Could you check a few things on this model? Use its own coordinates, in mm. A direction names the side the tool comes from. Round coordinates to 2 decimals unless told otherwise and drop trailing zeros. Order: outer loops, then holes, each group sorted by start corner. A loop starts at its lowest first (then second) coordinate and runs counter-clockwise, first axis right, second up. Notation, with made-up numbers: (-2, 7) -> (5, 7) arc R8 ccw to (5, 13) -> close; hole circle Ø1 at (4, -23.5). An arc over 180 degrees is marked (long way). Put each result on its own line as item: value. Start each with the question number.
from build123d import *

# Parameters (mm, degrees)
SKETCH2_R           = 3
BOSS_EXTRUDE1_DEPTH = 30


with BuildPart() as part:
    # Sketch1 → Revolve1 (revolve)
    with BuildSketch(Plane.XY):
        Polygon((0, 0), (10, 0), (10, 1), (5, 1), (5, 4), (10, 4), (10, 5), (0, 5), align=None)
    revolve(axis=Axis((0, 5, 0), (0, -1, 0)))

    # Sketch2 → Boss-Extrude1 (add)
    with BuildSketch(Plane(origin=(0, 5, 0), x_dir=(1, 0, 0), z_dir=(0, 1, 0))):
        Circle(SKETCH2_R)
    extrude(amount=BOSS_EXTRUDE1_DEPTH)


solid = part.part
1. For pin 1 Ø4 at (x, y) = (4, 16) entering from -Z; pin 2 Ø2 at (y, z) = (21.5, 0.5) entering from -X; pin 3 Ø4 at (y, z) = (18, 4.5) entering from +X, each with a flat end and sliding along its axis, tell me the tip position at first contact or that it passes through.
2. If we section it at A-A, the plane x = -8: Please give me the cut outline in (y, z).
3. Thinking about a two-plate mould opening in Y: for faces 4 (the face through (-2.17, 4.51, -9.76)), 5 (the face through (2, 1, 5)), 6 (the face through (0, 0, 0)), which applies, +Y half, -Y half, draft (parallel to the pull), parting line (faces both ways), or undercut?
4. I need wall thicknesses on L1, parallel to Y at x = 6.5, z = 3.75; L2, parallel to Y at x = 4, z = 1; L3, parallel to X at y = 21, z = -1.5. Which ranges of each line are inside material? Lowest first, please.
5. Which directions (+Z, -Z, +X, -X, +Y, -Y) give clear straight access to the entire face, cutting with the end or side of a thin tool? Please do faces 1 (the face through (-1.08, 2.52, -4.88)), 2 (the face through (0, 35, 0)), 3 (the face through (2.1, 5, 2.4)).
6. If we section it at D-D, the plane x = 0: Please give me the cut outline in (y, z), then the cut area to 3 significant figures.
7. If we section it at B-B, the plane z = -5.75: Please give me the cut outline in (x, y), then the cut area to 3 significant figures.
8. If we section it at C-C, the plane z = 0: Please give me the cut outline in (x, y), then the cut area to 3 significant figures.
Results below:
1. pin 1: z = -2.24
1. pin 2: x = -3
1. pin 3: x = 1.66
2. outline: (0, -6) -> (1, -6) -> (1, 6) -> (0, 6) -> close; (4, -6) -> (5, -6) -> (5, 6) -> (4, 6) -> close
3. face 4: draft
3. face 5: undercut
3. face 6: -Y half
4. L1: 0 to 1, 4 to 5
4. L2: 0 to 5
4. L3: -2.6 to 2.6
5. face 1: none
5. face 2: +Z, -Z, +X, -X, +Y
5. face 3: +Y
6. outline: (0, -10) -> (1, -10) -> (1, -5) -> (4, -5) -> (4, -10) -> (5, -10) -> (5, -3) -> (35, -3) -> (35, 3) -> (5, 3) -> (5, 10) -> (4, 10) -> (4, 5) -> (1, 5) -> (1, 10) -> (0, 10) -> close
6. area: 250 mm2
7. outline: (-8.18, 0) -> (8.18, 0) -> (8.18, 1) -> (-8.18, 1) -> close; (-8.18, 4) -> (8.18, 4) -> (8.18, 5) -> (-8.18, 5) -> close
7. area: 32.7 mm2
8. outline: (-10, 0) -> (10, 0) -> (10, 1) -> (5, 1) -> (5, 4) -> (10, 4) -> (10, 5) -> (3, 5) -> (3, 35) -> (-3, 35) -> (-3, 5) -> (-10, 5) -> (-10, 4) -> (-5, 4) -> (-5, 1) -> (-10, 1) -> close
8. area: 250 mm2
